Could you check a few things on this model? Use its own coordinates, in mm. Face numbers are marked on the shaded views. A direction names the side the tool comes from. Round coordinates to 2 decimals unless told otherwise and drop trailing zeros. Loops run counter-clockwise (first coordinate to the right, second up) from the corner with the lowest first, then second, coordinate; pieces in that order, holes last. Notation, with made-up numbers: M 30,78 L 59,78 A13 cw 59,91 Z; hole C 65,75.25 d3. An arc over 180 degrees is marked long. One line per item, written item: value. Start each with the question number.
Q1. I'm going to push flat-ended pins straight in: pin 1 Ø2 at (x, y) = (-0.5, 2.5) entering from +Z; pin 2 Ø2 at (y, z) = (2.5, -2) entering from -X; pin 3 Ø1.5 at (x, z) = (0.5, 1.5) entering from +Y. Where does each tip first touch, or does it pass through?
Q2. Thinking about a two-plate mould opening in Y: for the marked faces 1, 2 and 3, which applies, released by +Y, released by -Y, zero draft, split by the parting line, or undercut?
Q3. Imagine slicing it at A-A (x = 4.75). Please give me the cut outline in (y, z), then the cut area to 3 significant figures.
Q4. Which directions (+Z, -Z, +X, -X, +Y, -Y) give clear straight access to the entire face, cutting with the end or side of a thin tool? Please do the marked faces 4 and 5.
Q5. Please list where these lines run through material, in increasing order: line 1 along X through (y, z) = (0.5, -0.25); line 2 along Z through (x, y) = (-1.5, -0.25); line 3 along X through (y, z) = (2, -0.5).
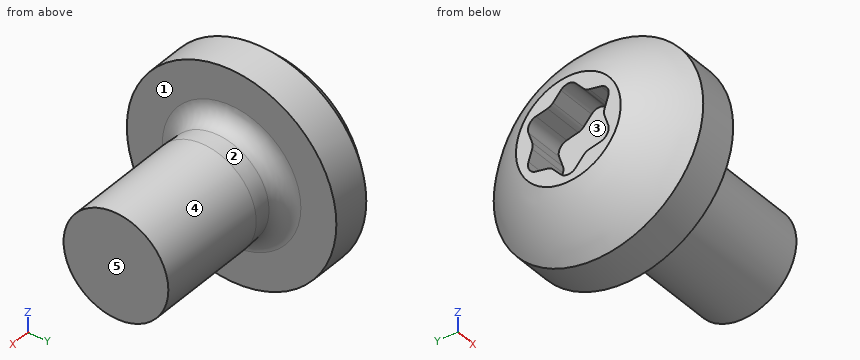
Autodesk Inventor part; units mm, degrees
ref_plane "YZ Plane" through (0, 0, 0) normal (1, 0, 0) x (0, 1, 0)
ref_plane "XZ Plane" through (0, 0, 0) normal (0, 1, 0) x (-1, 0, 0)
ref_plane "XY Plane" through (0, 0, 0) normal (0, 0, 1) x (1, 0, 0)
sketch "Sketch4" plane through (0, 0, 0) normal (0, 0, 1) x (1, 0, 0)
  line L0 (-2.6, 0) -> (5, 0)
  line L1 (0, 0) -> (-2.6, 0)
  line L2 (0, 3.5) -> (0, 2.315)
  line L3 (0.6, 1.715) -> (0.6, 1.715)
  line L4 (0.6, 1.715) -> (1.2, 1.75)
  arc A0 (0, 2.315) -> (0.6, 1.715) centre (0.6, 2.315) ccw
  line L5 (-2.6, 0) -> (-2.6, 1.75)
  line L6 (0, 3.5) -> (-1.2954, 3.5)
  arc A1 (-1.2954, 3.5) -> (-2.6, 1.75) centre (2.7825, -0.9012) ccw
  line L7 (1.2, 1.75) -> (5, 1.75)
  line L8 (5, 1.75) -> (5, 0)
  point P0 (0, 1.715)
  dimension "d71" = 0.6
  dimension "d72" = 5
  dimension "d74" = 0.6
  dimension "d75" = 3.43
  dimension "d78" = 3.5
  dimension "d82" = 6
  dimension "d83" = 2.6
  dimension "d84" = 7
  dimension "d104" = 3.8
  dimension "d105" = 3.5
revolve "Revolution7" add sketch "Sketch4" angle 360 about axis through (-2.6, 0, 0) along (1, 0, 0)
sketch "Sketch5" plane through (-2.6, 0, 0) normal (-1, 0, 0) x (0, 0, 1)
  circle A0 centre (0, 0) radius 1.675 construction
  circle A1 centre (0, 0) radius 1.1725 construction
  line L0 (0, 0) -> (-1.0154, 0.5862)
  line L1 (0, 0) -> (-1.0154, -0.5862)
  line L2 (-1.8008, 0) -> (1.7887, 0)
  line L3 (-1.675, 0) -> (-1.0154, -0.5862)
  line L4 (-1.675, 0) -> (-1.0154, 0.5862)
  point P0 (0, 0)
  dimension "d88" = 3.35
  dimension "d89" = 2.345
  dimension "d90" = 30
  dimension "d91" = 30
extrude "Extrusion1" cut sketch "Sketch5" against normal blind 1.33
pattern_circular "Circular Pattern1" count 6 over 360 about axis through (-10, 0, 0) along (1, 0, 0) of "Extrusion1"
fillet "Fillet1" radius 0.335 12 edges at (-1.935, -1.4506, -0.8375) (-1.935, -0.5862, -1.0154) (-1.935, -1.1725, 0) (-1.935, -1.4506, 0.8375) (-1.935, -0.5862, 1.0154) (-1.935, 0, 1.675) (-1.935, 1.1725, 0) (-1.935, 1.4506, 0.8375) (-1.935, 0.5863, 1.0154) (-1.935, 0.5862, -1.0154) (-1.935, 0, -1.675) (-1.935, 1.4506, -0.8375)
thread "Thread7"
equation "\"a\" = 1.2"
equation "\"b\" = 3.8"
equation "\"dk\" = 7"
equation "\"k\" = 2.6"
equation "\"r\" = 0.6"
equation "\"rf\" = 6"
equation "\"x\" = 0.6"
equation "\"A_\" = 3.35"
equation "\"t\" = 1.33"
equation "\"p\" = 0.6"
equation "\"l_\" = 5"
equation "\"d\" = 3.5"
equation "\"ds_\" = 3.43"
equation "\"lg\" = 0"
properties part number "Винты со звездообразным углублением в плоско-выпуклой головке ISO 14583 — M3,5 x 5 — 4.8" material "Сталь"
Report:
1. pin 1: stops at z = 3.16
1. pin 2: stops at x = -2.35
1. pin 3: stops at y = 3.37
2. face 1: zero draft
2. face 2: split by the parting line
2. face 3: undercut
3. outline: C 0,0 d3.5
3. area: 9.62 mm²
4. face 4: +X
4. face 5: +Z, -Z, +X, +Y, -Y
5. line 1: x = -1.27 to 5
5. line 2: z = -3.29 to -1.39, 1.39 to 3.29
5. line 3: x = -2.43 to 0.06
